The listing builds one solid part. Answer for the finished solid, in the listing's coordinates (mm). A direction names the side the tool comes from. Give positions to 0.01 mm unless a question says otherwise; leave off trailing zeros. Loops run counter-clockwise (first coordinate to the right, second up) from the corner with the lowest first, then second, coordinate; pieces in that order, holes last.
Item 1: A tool of negligible diameter and unlimited length cuts with its end or side. For faces 4 (the face through (3, 3, 0)), 5 (the face through (17.042, -4.769, -21.477)), 6 (the face through (9.92, 13.38, 25.73)), from which of +Z, -Z, +X, -X, +Y, -Y can it reach the whole face along a straight path? Write none if from no direction.
Item 2: Each of these flat-tipped pins is pushed along its axis until it touches: pin 1 Ø4 at (x, y) = (12, 8.5) entering from -Z; pin 2 Ø3 at (x, z) = (5.5, 2) entering from +Y; pin 3 Ø8 at (x, z) = (12, 9.5) entering from -Y. Where does it stop, or does it pass through?
Item 3: Section C-C, the plane x = 5.5 is taken. Give the vertices of the cut face in (y, z).
Item 4: Section B-B, the plane z = 0 is taken. Give the vertices of the cut face in (x, y).
Item 5: Section D-D, the plane x = 8.75 is taken. Give the vertices of the cut face in (y, z), and give its area (3 significant figures).
Item 6: The mould has two halves that part along Y. Classify faces 1 (the face through (0, -12, 0)), 2 (the face through (0.25, 25.245, -0.519)), 3 (the face through (14, -7, 18)): pulls with the +Y half, pulls with the -Y half, needs draft (parallel to the pull), parting line crosses it, or undercut.
Item 7: Section A-A, the plane y = 0 is taken. Give the vertices of the cut face in (x, z).
Item 8: Consider line 1 along Z through (x, y) = (16, 14); line 2 along Z through (x, y) = (16.75, 0); line 3 along Z through (x, y) = (17.9, 0). Determine where each line is inside the solid, lowest interval first.
Autodesk Inventor part; units mm, degrees
ref_plane "YZ Plane" through (0, 0, 0) normal (1, 0, 0) x (0, 1, 0)
ref_plane "XZ Plane" through (0, 0, 0) normal (0, 1, 0) x (-1, 0, 0)
ref_plane "XY Plane" through (0, 0, 0) normal (0, 0, 1) x (1, 0, 0)
sketch "Эскиз1" plane through (0, 0, 0) normal (0, 0, 1) x (1, 0, 0)
  line L0 (0, 0) -> (20, 0)
  line L1 (20, 0) -> (20, 25)
  line L2 (16, 29) -> (4, 29)
  line L3 (0, 25) -> (0, 0)
  line L4 (4, 29) -> (0, 25)
  line L5 (16, 29) -> (20, 25)
  point P0 (20, 29)
  point P1 (0, 29)
  dimension "d14" = 20
  dimension "d15" = 29
  dimension "d16" = 4
  dimension "d17" = 4
  dimension "d18" = 4
  dimension "d19" = 4
revolve "Вращение3" add sketch "Эскиз1" angle 360 about axis through (0, 0, 0) along (1, 0, 0)
sketch "Эскиз3" plane through (0, 0, 0) normal (0, 0, 1) x (1, 0, 0)
  line L0 (20, -25) -> (20, 25) construction
  line L1 (20, 0) -> (20, 22)
  line L2 (14, 22) -> (20, 22)
  line L3 (14, 22) -> (14, 19)
  line L4 (14, 19) -> (17, 19)
  line L5 (17, 19) -> (17, 0)
  line L6 (17, 0) -> (20, 0)
  point P0 (0, 0)
  dimension "d21" = 22
  dimension "d22" = 19
  dimension "d23" = 6
  dimension "d24" = 3
revolve "Вращение4" cut sketch "Эскиз3" angle 360 about axis through (17, 0, 0) along (1, 0, 0)
sketch "Эскиз4" plane through (0, 0, 0) normal (0, 0, 1) x (1, 0, 0)
  line L0 (0, -25) -> (0, 25) construction
  line L1 (0, 3) -> (7, 3)
  line L2 (7, 3) -> (7, -3)
  line L3 (7, -3) -> (0, -3)
  line L4 (0, -3) -> (0, 3)
  point P0 (0, 0)
  point P1 (0, 0)
  point P2 (0, 0)
  dimension "d26" = 7
  dimension "d27" = 6
extrude "Выдавливание1" cut sketch "Эскиз4" along normal through all both and the other way through all
properties part number "711127"
Worked answers:
1. face 4: +Z, -Z, -X
1. face 5: +X
1. face 6: +X, -X
2. pin 1: stops at z = -28.26
2. pin 2: stops at y = 29
2. pin 3: stops at y = -28.47
3. outline: (-3, -28.84) - (-3, 28.84) arc R29 ccw to start; (3, -28.84) arc R29 ccw to (3, 28.84) - close
4. outline: (0, -25) - (4, -29) - (16, -29) - (20, -25) - (20, -22) - (14, -22) - (14, -19) - (17, -19) - (17, 19) - (14, 19) - (14, 22) - (20, 22) - (20, 25) - (16, 29) - (4, 29) - (0, 25) - (0, 3) - (7, 3) - (7, -3) - (0, -3) - close
5. outline: circle Ø58 at (0, 0)
5. area: 2,640 mm2
6. face 1: needs draft
6. face 2: pulls with the +Y half
6. face 3: undercut
7. outline: (7, -29) - (16, -29) - (20, -25) - (20, -22) - (14, -22) - (14, -19) - (17, -19) - (17, 19) - (14, 19) - (14, 22) - (20, 22) - (20, 25) - (16, 29) - (7, 29) - close
8. line 1: z = -25.4 to -16.97, -12.85 to 12.85, 16.97 to 25.4
8. line 2: z = -28.25 to -22, -19 to 19, 22 to 28.25
8. line 3: z = -27.1 to -22, 22 to 27.1
